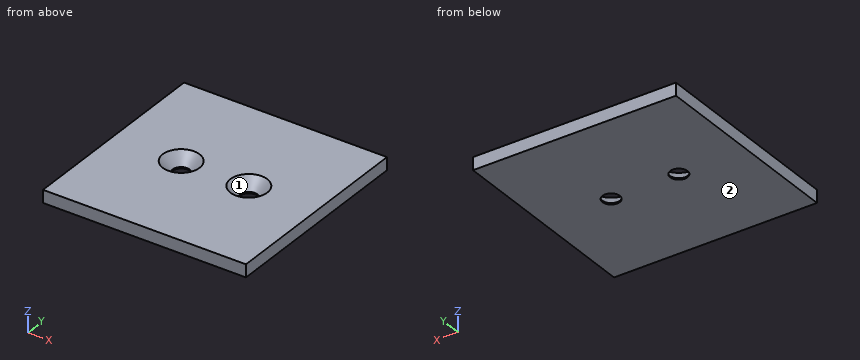
```python
from build123d import *

# Parameters (mm, degrees)
SKETCH1_W           = 76.2
SKETCH1_H           = 76.2
SKETCH1_R           = 3.2639
BOSS_EXTRUDE1_DEPTH = 2.38125


with BuildPart() as part:
    # Sketch1 → Boss-Extrude1 (new, symmetric)
    with BuildSketch(Plane.XY):
        Rectangle(SKETCH1_W, SKETCH1_H)
        with Locations(Location((-12.7, 0, 0), (0, 0, 180))):
            Circle(SKETCH1_R, mode=Mode.SUBTRACT)
        with Locations(Location((12.7, 0, 0), (0, 0, 180))):
            Circle(SKETCH1_R, mode=Mode.SUBTRACT)
    extrude(amount=BOSS_EXTRUDE1_DEPTH, both=True)

    # Sketch2 → Cut-Revolve1 (revolve, cut)
    with BuildSketch(Plane(origin=(0, 0, 0), x_dir=(1, 0, 0), z_dir=(0, 1, 0)), mode=Mode.PRIVATE) as cut_revolve1_sk:
        Polygon((-5.7658, -2.38125), (-12.7, 5.595634609), (-12.7, -2.38125), align=None)
    cut_revolve1 = revolve(cut_revolve1_sk.sketch.rotate(Axis((-12.7, 0, -5.595634609), (0, 0, 1)), 180), axis=Axis((-12.7, 0, -5.595634609), (0, 0, 1)), mode=Mode.SUBTRACT)

    # Sketch-Pattern1: Cut-Revolve1 at 1 more place
    with Locations((25.4, 0, 0)):
        add(cut_revolve1, mode=Mode.SUBTRACT)


solid = part.part
```
Geometry: final body of the model. Coordinates: model frame, mm. Face numbers are marked on the shaded views. Give positions to 0.01 mm unless a question says otherwise; leave off trailing zeros. Loops run counter-clockwise (first coordinate to the right, second up) from the corner with the lowest first, then second, coordinate; pieces in that order, holes last. Notation, with made-up numbers: (32, 2) - (73, 2) arc R18 ccw to (73, 21) - close; hole circle Ø9 at (78, 83). An arc over 180 degrees is marked (long way). Answer as CSV lines item,"result". Start each with the question number.
(1) Mould query, pull axis Y, two halves, no side actions, for the marked faces 1 and 2. Classes: +Y half, -Y half, draft (parallel to the pull), parting line (faces both ways), or undercut.
(2) Pin query (flat end, axial travel): P1, Ø8.5, axis at x = -12.7, y = 0, coming from the +Z side. Return the tip coordinate at first contact, or that it passes through.
(3) Section query B-B (x = -12.7). Output: boundary loops of the cut face in (y, z).
(4) Section query C-C (z = -0.5). Output: boundary loops of the cut face in (x, y), and give its area (3 significant figures).
(5) Section query A-A (y = 0). Output: boundary loops of the cut face in (x, z).
(6) Ray query, line 1 along Y through (x, z) = (12.7, -2); line 2 along Y through (x, z) = (10, 1.7); line 3 along X through (y, z) = (3, -0.15). Return the intervals inside material, ascending. Write a range as [from, to].
Worked answers:
1,face 1,"undercut"
1,face 2,"draft"
2,P1,"stops at z = -0.71"
3,outline,"(-38.1, -2.38) - (-3.26, -2.38) - (-3.26, -1.84) - (-6.93, 2.38) - (-38.1, 2.38) - close; (3.26, -2.38) - (38.1, -2.38) - (38.1, 2.38) - (6.93, 2.38) - (3.26, -1.84) - close"
4,outline,"(-38.1, -38.1) - (38.1, -38.1) - (38.1, 38.1) - (-38.1, 38.1) - close; hole circle Ø8.86 at (-12.7, 0); hole circle Ø8.86 at (12.7, 0)"
4,area,"5,680 mm^2"
5,outline,"(-38.1, -2.38) - (-15.96, -2.38) - (-15.96, -1.84) - (-19.63, 2.38) - (-38.1, 2.38) - close; (-9.44, -2.38) - (9.44, -2.38) - (9.44, -1.84) - (5.77, 2.38) - (-5.77, 2.38) - (-9.44, -1.84) - close; (15.96, -2.38) - (38.1, -2.38) - (38.1, 2.38) - (19.63, 2.38) - (15.96, -1.84) - close"
6,line 1,"y = [-38.1, -3.26], [3.26, 38.1]"
6,line 2,"y = [-38.1, -5.74], [5.74, 38.1]"
6,line 3,"x = [-38.1, -16.36], [-9.04, 9.04], [16.36, 38.1]"
